```python
from build123d import *

# Parameters (mm, degrees)
F1_DEPTH = 6.35
F3_D     = 8.7376
F4_R     = 12.7
F5_R     = 6.35


with BuildPart() as f1:
    # F0 (on Front) → F1 (new body)
    with BuildSketch(Plane.XZ):
        with BuildLine():
            Line((-141.7374620444, -81.8321618656), (-82.620901982, -47.7012))
            ThreePointArc((-82.620901982, -47.7012), (-75.6878127118, -58.0773013549), (-67.4596839815, -67.4596839815))
            Line((-67.4596839815, -67.4596839815), (-15.8232112853, -15.8232112853))
            ThreePointArc((-15.8232112853, -15.8232112853), (-20.6740218508, 8.5634602394), (0, 22.3774))
            Line((0, 22.3774), (0, 95.4024))
            ThreePointArc((0, 95.4024), (-71.1544614181, 63.5504566943), (-94.7963262761, -10.7365939814))
            Line((-94.7963262761, -10.7365939814), (-160.7874620444, -48.8365939814))
            Line((-160.7874620444, -48.8365939814), (-188.2837686146, -64.7115939814))
            Line((-188.2837686146, -64.7115939814), (-169.2337686146, -97.7071618656))
            Line((-169.2337686146, -97.7071618656), (-141.7374620444, -81.8321618656))
        make_face()
    extrude(amount=F1_DEPTH)

    # F3 (through all)
    with Locations(Plane.XZ.offset(6.35)):
        with Locations((-44.2468, 76.6377056723), (-76.6377056723, -44.2468)):
            Hole(F3_D / 2)

    # F4
    f4_edges = [f1.edges().sort_by_distance(p)[0] for p in [
        (-82.620902, -3.175, -47.7012),
        (-94.796326, -3.175, -10.736594),
    ]]
    fillet(f4_edges, radius=F4_R)

    # F5
    f5_edges = [f1.edges().sort_by_distance(p)[0] for p in [
        (-67.459684, -3.175, -67.459684),
        (-15.823211, -3.175, -15.823211),
        (0, -3.175, 22.3774),
        (0, -3.175, 95.4024),
    ]]
    fillet(f5_edges, radius=F5_R)


solid = f1.part
```
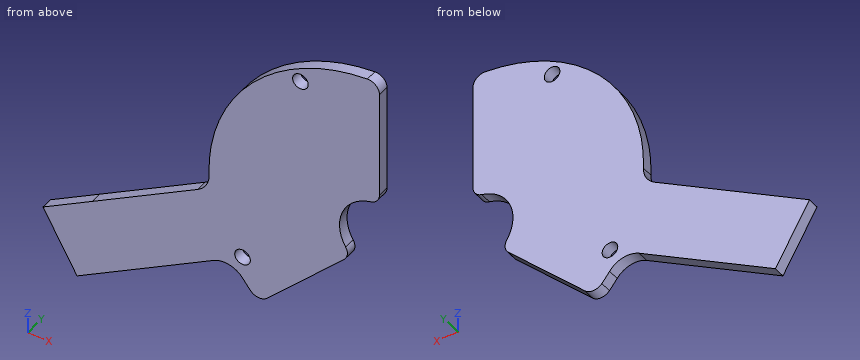
CAD build for the part. Positions are in the model's coordinates, mm. Coordinates: 2 decimals unless noted, no trailing zeros. Order: outer loops, then holes, each group sorted by start corner. A loop starts at its lowest first (then second) coordinate and runs counter-clockwise, first axis right, second up. Notation, with made-up numbers: (58.25, 57.25) - (87.25, 57.25) arc R18 cw to (87.25, 78.25) - close; hole circle Ø9 at (4.5, -37.5). An arc over 180 degrees is marked (long way). Answer in a Markdown table with one row per item.
1. Slice it at B-B, the plane x = -32. List the corners of the cut face in (y, z).
Answer:
| item | result |
|---|---|
| outline | (-6.35, -32) - (0, -32) - (0, 89.88) - (-6.35, 89.88) - close |
2. Flat gauge pins, fed straight in: P1, Ø8, axis at x = -44.25, z = 76.64, coming from the -Y side; P2, Ø2, axis at x = -120.5, y = -1.5, coming from the +Z side; P3, Ø2, axis at x = -157, y = -0.5, coming from the +Z side; P4, Ø1.5, axis at x = -65, y = -3, coming from the -Z side. Where does each tip first touch, or does it go through?
Answer:
| item | result |
|---|---|
| P1 | through |
| P2 | z = -25 |
| P3 | z = -46.07 |
| P4 | z = -64.48 |
3. Slice it at C-C, the plane z = 24. List the corners of the cut face in (x, y), then the cut area to 3 significant figures.
Answer:
| item | result |
|---|---|
| outline | (-92.33, -6.35) - (-1.43, -6.35) - (-1.43, 0) - (-92.33, 0) - close |
| area | 577 mm² |
4. Drill centre lines: L1, parallel to Z at x = -80, y = -2; L2, parallel to X at y = -6, z = 79; L3, parallel to X at y = -3, z = -53. Where is each one in solid material? Low to high. Write a range as from..to.
Answer:
| item | result |
|---|---|
| L1 | -53.84..-47.04, -41.46..51.98 |
| L2 | -53.48..-47.92, -40.57..0 |
| L3 | -168..-91.62, -81.62..-53 |
5. Slice it at A-A, the plane y = -2.25. List the corners of the cut face in (x, z), then the cut area to 3 significant figures.
Answer:
| item | result |
|---|---|
| outline | (-188.28, -64.71) - (-169.23, -97.71) - (-92.97, -53.68) arc R12.7 cw to (-76.44, -57.08) arc R95.4 ccw to (-72.1, -62.48) arc R6.35 ccw to (-62.81, -62.81) - (-19.81, -19.81) arc R6.35 ccw to (-18.93, -11.93) arc R22.38 cw to (-4.95, 21.82) arc R6.35 ccw to (0, 28.02) - (0, 88.83) arc R6.35 ccw to (-6.8, 95.16) arc R95.4 ccw to (-95.35, -3.28) arc R12.7 cw to (-101.69, -14.72) - close; hole circle Ø8.74 at (-76.64, -44.25); hole circle Ø8.74 at (-44.25, 76.64) |
| area | 13,900 mm² |
